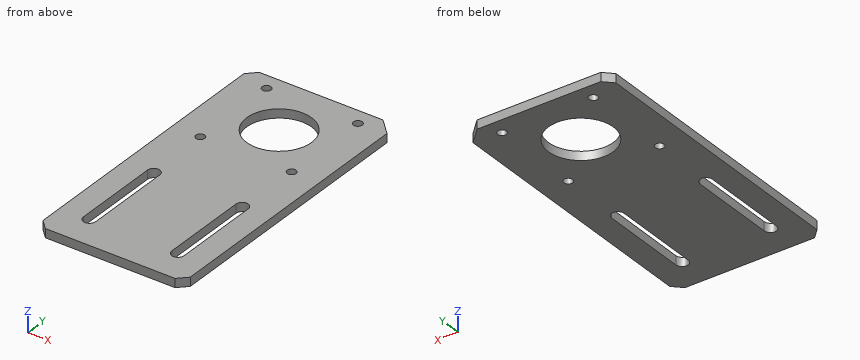
from build123d import *

# Parameters (mm, degrees)
SKETCH_1_R      = 1.5
SKETCH_1_R_2    = 11
EXTRUDE_1_DEPTH = 3
CHAMFER_1_SIZE  = 3


with BuildPart() as part:
    # 草图1 → 凸台-拉伸1 (new body)
    with BuildSketch(Plane.XY):
        Polygon((45, 0), (50, -5), (50, -100), (0, -100), (0, 0), align=None)
        with Locations((9.5, -36.5)):
            Circle(SKETCH_1_R, mode=Mode.SUBTRACT)
        with Locations((9.5, -5.5)):
            Circle(SKETCH_1_R, mode=Mode.SUBTRACT)
        with Locations((25, -21)):
            Circle(SKETCH_1_R_2, mode=Mode.SUBTRACT)
        with Locations((40.5, -36.5)):
            Circle(SKETCH_1_R, mode=Mode.SUBTRACT)
        with Locations((40.5, -5.5)):
            Circle(SKETCH_1_R, mode=Mode.SUBTRACT)
        with BuildLine():
            ThreePointArc((42.1, -59), (40, -56.9), (37.9, -59))
            Line((37.9, -59), (37.9, -89))
            ThreePointArc((37.9, -89), (40, -91.1), (42.1, -89))
            Line((42.1, -89), (42.1, -59))
        make_face(mode=Mode.SUBTRACT)
        with BuildLine():
            ThreePointArc((7.9, -89), (10, -91.1), (12.1, -89))
            Line((12.1, -89), (12.1, -59))
            ThreePointArc((12.1, -59), (10, -56.9), (7.9, -59))
            Line((7.9, -59), (7.9, -89))
        make_face(mode=Mode.SUBTRACT)
    extrude(amount=EXTRUDE_1_DEPTH)

    # 倒角1
    chamfer_1_edges = [part.edges().sort_by_distance(p)[0] for p in [
        (50, -100, 1.5),
        (0, -100, 1.5),
        (0, 0, 1.5),
    ]]
    chamfer(chamfer_1_edges, length=CHAMFER_1_SIZE)


solid = part.part
The listing builds one solid part. Answer for the finished solid, in the listing's coordinates (mm). Round coordinates to 2 decimals unless told otherwise and drop trailing zeros. Order: outer loops, then holes, each group sorted by start corner. A loop starts at its lowest first (then second) coordinate and runs counter-clockwise, first axis right, second up. Notation, with made-up numbers: M 65.5,-21 L 102.5,-21 A12 ccw 102.5,-8 Z; hole C 0,-0.5 d9. An arc over 180 degrees is marked long. Answer in a Markdown table with one row per item. Add a question column.
1) Consider line 1 along X through (y, z) = (-88, 0.45); line 2 along Y through (x, z) = (25, 1.75); line 3 along Y through (x, z) = (10, 0.45). Determine where each line is inside the solid, lowest interval first. Write a range as from..to.
2) The part is cut by section A-A on y = -83.5. Determine the outline of the cut face in (x, z), plus the area to 3 significant figures.
3) The part is cut by section C-C on x = 20.5. Determine the outline of the cut face in (y, z).
4) The part is cut by section B-B on z = 1.8. Determine the outline of the cut face in (x, y).
5) A flat-ended cylindrical pin translates along its axis: pin 1 Ø2.5 at (x, y) = (40.5, -5.5) entering from +Z. Find the tip coordinate at first contact, or state that the pin passes through.
6) The part is cut by section D-D on y = -36.5. Determine the outline of the cut face in (x, z), plus the area to 3 significant figures.
Findings below:
| question | item | result |
|---|---|---|
| 1 | line 1 | x = 0..7.9, 12.1..37.9, 42.1..50 |
| 1 | line 2 | y = -100..-32, -10..0 |
| 1 | line 3 | y = -100..-91.1, -56.9..-37.91, -35.09..-6.91, -4.09..0 |
| 2 | outline | M 0,0 L 7.9,0 L 7.9,3 L 0,3 Z; M 12.1,0 L 37.9,0 L 37.9,3 L 12.1,3 Z; M 42.1,0 L 50,0 L 50,3 L 42.1,3 Z |
| 2 | area | 125 mm² |
| 3 | outline | M -100,0 L -31.04,0 L -31.04,3 L -100,3 Z; M -10.96,0 L 0,0 L 0,3 L -10.96,3 Z |
| 4 | outline | M 0,-97 L 3,-100 L 47,-100 L 50,-97 L 50,-5 L 45,0 L 3,0 L 0,-3 Z; hole M 7.9,-89 A2.1 ccw 12.1,-89 L 12.1,-59 A2.1 ccw 7.9,-59 Z; hole C 9.5,-36.5 d3; hole C 9.5,-5.5 d3; hole C 25,-21 d22; hole M 37.9,-89 A2.1 ccw 42.1,-89 L 42.1,-59 A2.1 ccw 37.9,-59 Z; hole C 40.5,-36.5 d3; hole C 40.5,-5.5 d3 |
| 5 | pin 1 | passes through |
| 6 | outline | M 0,0 L 8,0 L 8,3 L 0,3 Z; M 11,0 L 39,0 L 39,3 L 11,3 Z; M 42,0 L 50,0 L 50,3 L 42,3 Z |
| 6 | area | 132 mm² |
